Input: part model. Units: mm. Frame: model coordinates. Coordinates: 2 decimals unless noted, no trailing zeros. Order: outer loops, then holes, each group sorted by start corner. A loop starts at its lowest first (then second) coordinate and runs counter-clockwise, first axis right, second up.
from build123d import *

# Parameters (mm, degrees)
F0_R     = 10
F0_R_2   = 5.4110615761
F1_DEPTH = 25
F2_DEPTH = 25


with BuildPart() as f1:
    # F0 (on Top) → F1 (new body)
    with BuildSketch(Plane.XY):
        with BuildLine():
            Line((-56.9581672003, 45.2024476719), (-15.9581672003, 45.2024476719))
            ThreePointArc((-15.9581672003, 45.2024476719), (-28.3942012079, 78.2016667372), (-59.5161055572, 94.7857093817))
            ThreePointArc((-59.5161055572, 94.7857093817), (-69.1375376467, 99.0362543602), (-78.191763881, 93.6827437957))
            ThreePointArc((-78.191763881, 93.6827437957), (-115.5981273519, 51.1919681993), (-89.3719782194, 1.0233411444))
            ThreePointArc((-89.3719782194, 1.0233411444), (-102.1550099365, -77.6490774294), (-22.9581672003, -68.6704670274))
            ThreePointArc((-22.9581672003, -68.6704670274), (-17.7399133953, -56.3845219384), (-15.9581672003, -43.1557653831))
            Line((-15.9581672003, -43.1557653831), (-56.9581672003, -43.1557653831))
            ThreePointArc((-56.9581672003, -43.1557653831), (-63.322128231, -40.5197264137), (-65.9581672003, -34.1557653831))
            Line((-65.9581672003, -34.1557653831), (-65.9581672003, 36.2024476719))
            ThreePointArc((-65.9581672003, 36.2024476719), (-63.322128231, 42.5664087025), (-56.9581672003, 45.2024476719))
        make_face()
        with Locations((-76.8970996141, -56.245483458)):
            Circle(F0_R, mode=Mode.SUBTRACT)
        with BuildLine():
            Line((25.0418327997, 45.2024476719), (-15.9581672003, 45.2024476719))
            Line((-15.9581672003, 45.2024476719), (-56.9581672003, 45.2024476719))
            ThreePointArc((-56.9581672003, 45.2024476719), (-63.322128231, 42.5664087025), (-65.9581672003, 36.2024476719))
            Line((-65.9581672003, 36.2024476719), (-65.9581672003, -34.1557653831))
            ThreePointArc((-65.9581672003, -34.1557653831), (-63.322128231, -40.5197264137), (-56.9581672003, -43.1557653831))
            Line((-56.9581672003, -43.1557653831), (-15.9581672003, -43.1557653831))
            Line((-15.9581672003, -43.1557653831), (25.0418327997, -43.1557653831))
            ThreePointArc((25.0418327997, -43.1557653831), (31.4057938304, -40.5197264137), (34.0418327997, -34.1557653831))
            Line((34.0418327997, -34.1557653831), (34.0418327997, 36.2024476719))
            ThreePointArc((34.0418327997, 36.2024476719), (31.4057938304, 42.5664087025), (25.0418327997, 45.2024476719))
        make_face()
        with BuildLine():
            ThreePointArc((25.7441905011, 94.5091321303), (-4.1346135706, 77.4911290097), (-15.9581672003, 45.2024476719))
            Line((-15.9581672003, 45.2024476719), (25.0418327997, 45.2024476719))
            ThreePointArc((25.0418327997, 45.2024476719), (31.4057938304, 42.5664087025), (34.0418327997, 36.2024476719))
            Line((34.0418327997, 36.2024476719), (34.0418327997, -34.1557653831))
            ThreePointArc((34.0418327997, -34.1557653831), (31.4057938304, -40.5197264137), (25.0418327997, -43.1557653831))
            Line((25.0418327997, -43.1557653831), (-15.9581672003, -43.1557653831))
            ThreePointArc((-15.9581672003, -43.1557653831), (-14.1764210053, -56.3845219384), (-8.9581672003, -68.6704670274))
            ThreePointArc((-8.9581672003, -68.6704670274), (70.2386755359, -77.6490774294), (57.4556438187, 1.0233411444))
            ThreePointArc((57.4556438187, 1.0233411444), (83.6067922706, 51.7838451407), (45.1150959261, 93.9608607278))
            ThreePointArc((45.1150959261, 93.9608607278), (35.5797605926, 99.5387739728), (25.7441905011, 94.5091321303))
        make_face()
        with Locations((45.5559305847, -56.245483458)):
            Circle(F0_R, mode=Mode.SUBTRACT)
        with BuildLine():
            ThreePointArc((-15.9581672003, -43.1557653831), (-17.7399133953, -56.3845219384), (-22.9581672003, -68.6704670274))
            Line((-22.9581672003, -68.6704670274), (-22.9581672003, -234.5025837421))
            Line((-22.9581672003, -234.5025837421), (-22.9581672003, -380.6582093239))
            Line((-22.9581672003, -380.6582093239), (-8.9581672003, -380.6582093239))
            Line((-8.9581672003, -380.6582093239), (-8.9581672003, -234.5025837421))
            Line((-8.9581672003, -234.5025837421), (-8.9581672003, -68.6704670274))
            ThreePointArc((-8.9581672003, -68.6704670274), (-14.1764210053, -56.3845219384), (-15.9581672003, -43.1557653831))
        make_face()
        with Locations((-15.9581672003, -356.8059802055)):
            Circle(F0_R_2, mode=Mode.SUBTRACT)
    extrude(amount=F1_DEPTH)

    # F0 (on Top) → F2 (join)
    with BuildSketch(Plane.XY):
        with BuildLine():
            Line((-56.9581672003, 45.2024476719), (-15.9581672003, 45.2024476719))
            ThreePointArc((-15.9581672003, 45.2024476719), (-28.3942012079, 78.2016667372), (-59.5161055572, 94.7857093817))
            ThreePointArc((-59.5161055572, 94.7857093817), (-69.1375376467, 99.0362543602), (-78.191763881, 93.6827437957))
            ThreePointArc((-78.191763881, 93.6827437957), (-115.5981273519, 51.1919681993), (-89.3719782194, 1.0233411444))
            ThreePointArc((-89.3719782194, 1.0233411444), (-102.1550099365, -77.6490774294), (-22.9581672003, -68.6704670274))
            ThreePointArc((-22.9581672003, -68.6704670274), (-17.7399133953, -56.3845219384), (-15.9581672003, -43.1557653831))
            Line((-15.9581672003, -43.1557653831), (-56.9581672003, -43.1557653831))
            ThreePointArc((-56.9581672003, -43.1557653831), (-63.322128231, -40.5197264137), (-65.9581672003, -34.1557653831))
            Line((-65.9581672003, -34.1557653831), (-65.9581672003, 36.2024476719))
            ThreePointArc((-65.9581672003, 36.2024476719), (-63.322128231, 42.5664087025), (-56.9581672003, 45.2024476719))
        make_face()
        with Locations((-76.8970996141, -56.245483458)):
            Circle(F0_R, mode=Mode.SUBTRACT)
        with BuildLine():
            Line((25.0418327997, 45.2024476719), (-15.9581672003, 45.2024476719))
            Line((-15.9581672003, 45.2024476719), (-56.9581672003, 45.2024476719))
            ThreePointArc((-56.9581672003, 45.2024476719), (-63.322128231, 42.5664087025), (-65.9581672003, 36.2024476719))
            Line((-65.9581672003, 36.2024476719), (-65.9581672003, -34.1557653831))
            ThreePointArc((-65.9581672003, -34.1557653831), (-63.322128231, -40.5197264137), (-56.9581672003, -43.1557653831))
            Line((-56.9581672003, -43.1557653831), (-15.9581672003, -43.1557653831))
            Line((-15.9581672003, -43.1557653831), (25.0418327997, -43.1557653831))
            ThreePointArc((25.0418327997, -43.1557653831), (31.4057938304, -40.5197264137), (34.0418327997, -34.1557653831))
            Line((34.0418327997, -34.1557653831), (34.0418327997, 36.2024476719))
            ThreePointArc((34.0418327997, 36.2024476719), (31.4057938304, 42.5664087025), (25.0418327997, 45.2024476719))
        make_face()
        with BuildLine():
            ThreePointArc((25.7441905011, 94.5091321303), (-4.1346135706, 77.4911290097), (-15.9581672003, 45.2024476719))
            Line((-15.9581672003, 45.2024476719), (25.0418327997, 45.2024476719))
            ThreePointArc((25.0418327997, 45.2024476719), (31.4057938304, 42.5664087025), (34.0418327997, 36.2024476719))
            Line((34.0418327997, 36.2024476719), (34.0418327997, -34.1557653831))
            ThreePointArc((34.0418327997, -34.1557653831), (31.4057938304, -40.5197264137), (25.0418327997, -43.1557653831))
            Line((25.0418327997, -43.1557653831), (-15.9581672003, -43.1557653831))
            ThreePointArc((-15.9581672003, -43.1557653831), (-14.1764210053, -56.3845219384), (-8.9581672003, -68.6704670274))
            ThreePointArc((-8.9581672003, -68.6704670274), (70.2386755359, -77.6490774294), (57.4556438187, 1.0233411444))
            ThreePointArc((57.4556438187, 1.0233411444), (83.6067922706, 51.7838451407), (45.1150959261, 93.9608607278))
            ThreePointArc((45.1150959261, 93.9608607278), (35.5797605926, 99.5387739728), (25.7441905011, 94.5091321303))
        make_face()
        with Locations((45.5559305847, -56.245483458)):
            Circle(F0_R, mode=Mode.SUBTRACT)
        with BuildLine():
            ThreePointArc((-15.9581672003, -43.1557653831), (-17.7399133953, -56.3845219384), (-22.9581672003, -68.6704670274))
            Line((-22.9581672003, -68.6704670274), (-22.9581672003, -234.5025837421))
            Line((-22.9581672003, -234.5025837421), (-22.9581672003, -380.6582093239))
            Line((-22.9581672003, -380.6582093239), (-8.9581672003, -380.6582093239))
            Line((-8.9581672003, -380.6582093239), (-8.9581672003, -234.5025837421))
            Line((-8.9581672003, -234.5025837421), (-8.9581672003, -68.6704670274))
            ThreePointArc((-8.9581672003, -68.6704670274), (-14.1764210053, -56.3845219384), (-15.9581672003, -43.1557653831))
        make_face()
        with Locations((-15.9581672003, -356.8059802055)):
            Circle(F0_R_2, mode=Mode.SUBTRACT)
    extrude(amount=F2_DEPTH)


solid = f1.part
Item 1: Cut plane D-D on x = -51. Return loops of the section in (y, z).
Response values:
outline: (-90.87, 0) - (92.91, 0) - (92.91, 25) - (-90.87, 25) - close
Item 2: Ray query, probe 1 along X at (y, z) = (-71.5, 4.75); probe 2 along X at (y, z) = (-62, 14); probe 3 along X at (y, z) = (-160, 22.5). Return the intervals inside material, ascending.
Response values:
probe 1: x = -107.15 to -24.77, -22.96 to -8.96, -7.15 to 75.23
probe 2: x = -112.27 to -85.08, -68.72 to 37.38, 53.73 to 80.35
probe 3: x = -22.96 to -8.96
Item 3: Draft query along Y for faces 1 (the face through (-115.49, 52.03, 12.32)), 2 (the face through (35.741, 99.533, 12.325)), 3 (the face through (-17, -30, 25)). Return one class per face: pulls with the +Y half, pulls with the -Y half, needs draft (parallel to the pull), parting line crosses it, or undercut.
Response values:
face 1: undercut
face 2: pulls with the +Y half
face 3: needs draft
Item 4: Cut plane A-A on y = 59.5. Return loops of the section in (x, z), then the cut area to 3 significant figures.
Response values:
outline: (-113.87, 0) - (-18.05, 0) - (-18.05, 25) - (-113.87, 25) - close; (-13.87, 0) - (81.95, 0) - (81.95, 25) - (-13.87, 25) - close
area: 4,790 mm2
Item 5: Cut plane B-B on y = -87. Return loops of the section in (x, z).
Response values:
outline: (-89.99, 0) - (-41.92, 0) - (-41.92, 25) - (-89.99, 25) - close; (-22.96, 0) - (-8.96, 0) - (-8.96, 25) - (-22.96, 25) - close; (10.01, 0) - (58.08, 0) - (58.08, 25) - (10.01, 25) - close
Item 6: Pin query (flat end, axial travel): pin 1 Ø12 at (x, z) = (-44, 21) entering from +Y; pin 2 Ø2 at (x, z) = (51, 12) entering from -Y; pin 3 Ø5 at (x, z) = (39, 20.5) entering from -Y. Return the tip coordinate at first contact, or that it passes through.
Response values:
pin 1: stops at y = 92.59
pin 2: stops at y = -90.54
pin 3: stops at y = -93.1
Item 7: Cut plane C-C on z = 16. Return loops of the section in (x, y).
Response values:
outline: (-89.37, 1.02) arc R50 ccw (long way) to (-22.96, -68.67) - (-22.96, -380.66) - (-8.96, -380.66) - (-8.96, -68.67) arc R50 ccw (long way) to (57.46, 1.02) arc R50 ccw to (45.12, 93.96) arc R11.5 ccw to (25.74, 94.51) arc R50 ccw to (-15.96, 45.2) arc R50 ccw to (-59.52, 94.79) arc R11.5 ccw to (-78.19, 93.68) arc R50 ccw to start; hole circle Ø20 at (-76.9, -56.25); hole circle Ø10.82 at (-15.96, -356.81); hole circle Ø20 at (45.56, -56.25)
